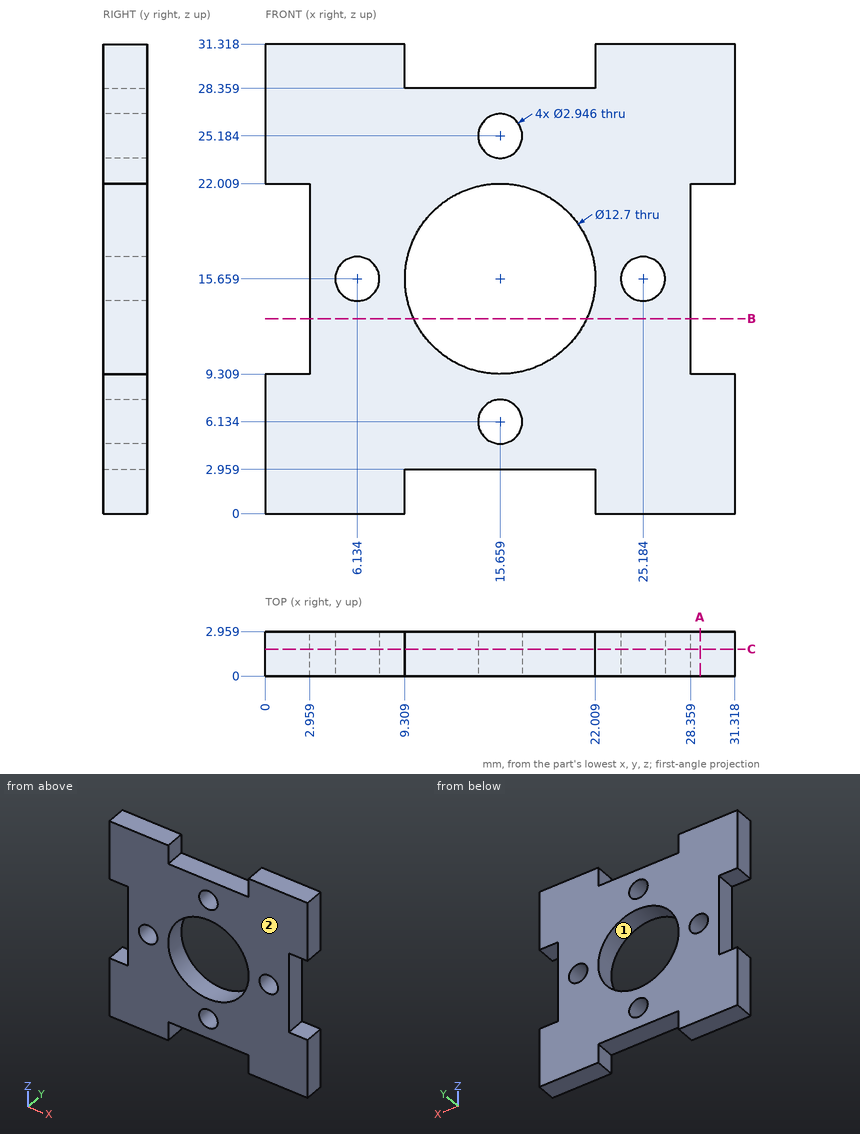
Design review of the part shown in the three views and the two pictorial views. Dimensions are in mm from the part's minimum x, y and z. Give positions to 0.01 mm unless a question says otherwise; leave off trailing zeros. Loops run counter-clockwise (first coordinate to the right, second up) from the corner with the lowest first, then second, coordinate; pieces in that order, holes last. Notation, with made-up numbers: M 8,-38.75 L 61,-38.75 A19 ccw 61,-29.75 Z; hole C 13,19 d2. An arc over 180 degrees is marked long. Answer as a JSON object with one key per item and string values. Group by question number.
Q1. For probe 1 along X at (y, z) = (0.7, 29.5); probe 2 along X at (y, z) = (0.75, 14.5) (1 decimal); probe 3 along X at (y, z) = (1.55, 5.5), list the stretches that pass through material, from the lowest coordinate up. Write a range as [from, to].
Q2. Add section C-C on y = 1.8. Give the boundary of the cut face in (x, z).
Q3. Insertion check: P1, Ø1, axis at x = 12, y = 1.5, coming from the +Z side; P2, Ø0.9, axis at y = 2, z = 30.5, coming from the -X side; P3, Ø1.5, axis at x = 15, y = 1, coming from the -Z side. Each pin has a flat end and moves straight along its axis. Give the tip position at first contact, or say it passes through.
Q4. Mouldability with a two-part tool opening along Z and no side actions: class the marked faces 1 and 2 as +Z half, -Z half, draft (parallel to the pull), parting line (faces both ways), or undercut.
Q5. Add section B-B on z = 13. Give the boundary of the cut face in (x, y) (1 decimal).
Q6. Add section A-A on x = 29. Give the boundary of the cut face in (y, z), and give its area (3 significant figures).
Checked values:
{
 "1": {"probe 1": "[0, 9.31], [22.01, 31.32]", "probe 2": "[3, 5.2], [7, 9.4], [21.9, 24.3], [26.1, 28.4]", "probe 3": "[0, 14.33], [16.99, 31.32]"},
 "2": {"outline": "M 0,0 L 9.31,0 L 9.31,2.96 L 22.01,2.96 L 22.01,0 L 31.32,0 L 31.32,9.31 L 28.36,9.31 L 28.36,22.01 L 31.32,22.01 L 31.32,31.32 L 22.01,31.32 L 22.01,28.36 L 9.31,28.36 L 9.31,31.32 L 0,31.32 L 0,22.01 L 2.96,22.01 L 2.96,9.31 L 0,9.31 Z; hole C 6.13,15.66 d2.95; hole C 15.66,15.66 d12.7; hole C 15.66,6.13 d2.95; hole C 15.66,25.18 d2.95; hole C 25.18,15.66 d2.95"},
 "3": {"P1": "z = 28.36", "P2": "x = 0", "P3": "z = 2.96"},
 "4": {"face 1": "undercut", "face 2": "draft"},
 "5": {"outline": "M 3,0 L 9.9,0 L 9.9,3 L 3,3 Z; M 21.4,0 L 28.4,0 L 28.4,3 L 21.4,3 Z"},
 "6": {"outline": "M 0,0 L 2.96,0 L 2.96,9.31 L 0,9.31 Z; M 0,22.01 L 2.96,22.01 L 2.96,31.32 L 0,31.32 Z", "area": "55.1 mm²"}
}
